Input: part model. Units: mm. Frame: model coordinates. Face numbers are marked on the shaded views. A direction names the side the tool comes from. Coordinates: 2 decimals unless noted, no trailing zeros. Write each loop counter-clockwise with the first axis right and the second up, starting at its lowest first coordinate (ties: lowest second). Pieces come first, ordered by that corner, then holes.
from build123d import *

# Parameters (mm, degrees)
CHAMFER_1_SIZE  = 0.5
CHAMFER_2_SIZE  = 0.6
CHAMFER_2_SIZE2 = 1.648486452


with BuildPart() as part:
    # Эскиз1 → Повернуть1 (revolve)
    with BuildSketch(Plane(origin=(0, 0, 0), x_dir=(0, 0, -1), z_dir=(1, 0, 0))):
        Polygon((0, 5.5), (7.8, 5.5), (7.8, 6.95), (3.265574507, 6.95), (3, 7), (1, 7), (1, 8), (0, 8), align=None)
    revolve(axis=Axis((0, 0, 0), (0, 0, -1)))

    # Фаска1
    chamfer_1_edges = [part.edges().sort_by_distance(p)[0] for p in [
        (0, -5.5, -7.8),
    ]]
    chamfer(chamfer_1_edges, length=CHAMFER_1_SIZE)

    # Фаска2
    chamfer_2_edges = [part.edges().sort_by_distance(p)[0] for p in [
        (0, -5.5, 0),
    ]]
    chamfer_2_side = [part.faces().sort_by_distance(p)[0] for p in [
        (0, -7.77372583, 0),
    ]]
    chamfer(chamfer_2_edges, length=CHAMFER_2_SIZE, length2=CHAMFER_2_SIZE2, reference=chamfer_2_side[0])


solid = part.part
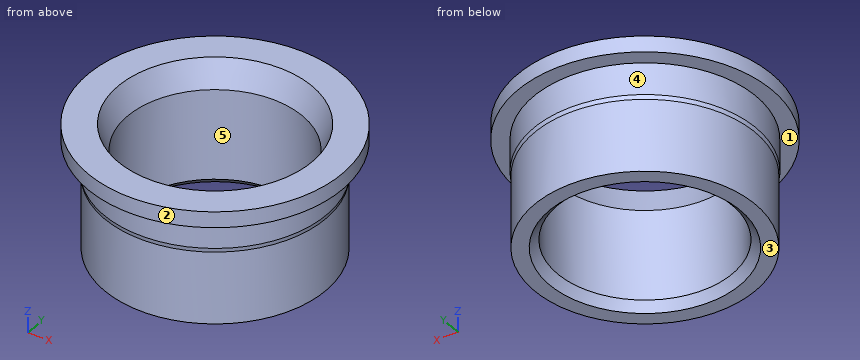
Item 1: Section query D-D, the plane z = -4.25. Return loops of the section in (x, y), then the cut area to 3 significant figures.
Item 2: Section query A-A, the plane y = 0. Return loops of the section in (x, z), then the cut area to 3 significant figures.
Item 3: Pull-direction query (Y, two-part tool) for the marked faces 3, 4 and 5; classes: released by +Y, released by -Y, zero draft, split by the parting line, or undercut.
Item 4: Pin query (flat end, axial travel): pin 1 Ø4 at (x, z) = (-2.5, -6) entering from +Y; pin 2 Ø3 at (y, z) = (2.5, -6.5) entering from +X; pin 3 Ø3 at (y, z) = (2, -4.5) entering from -X. Return the tip coordinate at first contact, or that it passes through.
Item 5: Section query C-C, the plane z = -2. Return loops of the section in (x, y).
Item 6: Material intervals for line 1 (X direction, y = 0, z = -5.5); line 2 (Y direction, x = 5, z = -2.25); line 3 (Y direction, x = -0.75, z = -0.25), sorted ascending.
Item 7: Access query for the marked faces 1 and 2. Directions: +Z, -Z, +X, -X, +Y, -Y. A direction counts if a zero-diameter tool reaches every point of the face in a straight line with its end or side. Return the directions, or none.
The answers:
1. outline: circle Ø13.9 at (0, 0); hole circle Ø11 at (0, 0)
1. area: 56.7 mm2
2. outline: (-8, -1) - (-7, -1) - (-7, -3) - (-6.95, -3.27) - (-6.95, -7.8) - (-6, -7.8) - (-5.5, -7.3) - (-5.5, -1.65) - (-6.1, 0) - (-8, 0) - close; (5.5, -7.3) - (6, -7.8) - (6.95, -7.8) - (6.95, -3.27) - (7, -3) - (7, -1) - (8, -1) - (8, 0) - (6.1, 0) - (5.5, -1.65) - close
2. area: 23.7 mm2
3. face 3: zero draft
3. face 4: split by the parting line
3. face 5: undercut
4. pin 1: stops at y = 6.93
4. pin 2: stops at x = 6.88
4. pin 3: stops at x = -6.93
5. outline: circle Ø14 at (0, 0); hole circle Ø11 at (0, 0)
6. line 1: x = -6.95 to -5.5, 5.5 to 6.95
6. line 2: y = -4.9 to -2.29, 2.29 to 4.9
6. line 3: y = -7.96 to -5.96, 5.96 to 7.96
7. face 1: -Z
7. face 2: +Z, -Z
